Source: CAD feature listing. Evaluate the final solid. Frame: model axes, mm. A direction names the side the tool comes from. Coordinates: 2 decimals unless noted, no trailing zeros. Order: outer loops, then holes, each group sorted by start corner. A loop starts at its lowest first (then second) coordinate and runs counter-clockwise, first axis right, second up. Notation, with made-up numbers: (80.5, 41) - (102.5, 41) arc R12 ccw to (102.5, 45) - close; hole circle Ø4 at (-29.5, -17.75). An arc over 180 degrees is marked (long way). One line per question, with ' | ' between items. Start each with the question number.
(1) Access query for faces 4 (the flat face through (185, -10, -69.85)), 5 (the flat face through (-148, 44, -50.8)), 6 (the flat face through (185, -10, 120.65)), 7 (the flat face through (-4, 0, -2)). Directions: +Z, -Z, +X, -X, +Y, -Y. A direction counts if a zero-diameter tool reaches every point of the face in a straight line with its end or side. Return the directions, or none.
(2) Section D-D (z = -1). Return the cut outline in (x, y).
(3) Section A-A (x = -103). Return the cut outline in (y, z), then the cut area to 3 significant figures.
(4) Contact query for flat-ended pins moving along their axis: P1, Ø20.5, axis at x = -181.5, y = -13.5, coming from the -Z side; P2, Ø6.5, axis at y = 43.5, z = 3.5, coming from the -X side; P3, Ø2, axis at x = -176.5, z = 96.5, coming from the -Y side. Output: stop coordinate, or through.
(5) Section B-B (z = -88). Return the cut outline in (x, y), then the cut area to 3 significant figures.
(6) Draft query along Y for faces 1 (the cylindrical face through (-184.974, -25.395, -94.894)), 2 (the flat face through (-25.4, 45, -1)), 3 (the flat face through (-185, -10, 69.85)). Return one class per face: +Y half, -Y half, draft (parallel to the pull), parting line (faces both ways), or undercut.
(7) Line query: line 1 along Y through (x, z) = (-208, 36); line 2 along Y through (x, z) = (-63, -69.5); line 3 along Z through (x, y) = (-187.5, -12.5). Output: solid intervals per line, ascending.
(8) Section C-C (x = 210). Return the cut outline in (y, z).
from build123d import *

# Parameters (mm, degrees)
CHASIS_W                = 533.4
CHASIS_H                = 279.4
BOSS_EXTRUDE1_DEPTH     = 152.4
SKETCH3_W               = 63.5
SKETCH3_H               = 50.8
MIRROR2_COPY_1_SKETCH_W = 63.5
MIRROR2_COPY_1_SKETCH_H = 50.8
SKETCH4_W               = 101.6
SKETCH4_H               = 12.7
CUT_EXTRUDE1_DEPTH      = 241.3


with BuildPart() as part:
    # Chasis → Boss-Extrude1 (new body)
    with BuildSketch(Plane(origin=(0, 0, 0), x_dir=(1, 0, 0), z_dir=(0, 1, 0))):
        Rectangle(CHASIS_W, CHASIS_H)
    extrude(amount=BOSS_EXTRUDE1_DEPTH)

    # Sketch3 → Revolve2 (revolve)
    with BuildSketch(Plane(origin=(0, 38.1, 0), x_dir=(-1, 0, 0), z_dir=(0, -1, 0))):
        with Locations((215.9, -95.25)):
            Rectangle(SKETCH3_W, SKETCH3_H)
    revolve2 = revolve(axis=Axis((-184.15, 38.1, 69.85), (0, 0, 1)))

    # Mirror1: Revolve2 across plane
    add(revolve2.mirror(Plane.XY))

    # Mirror2: Revolve2 across plane
    add(revolve2.mirror(Plane(origin=(0, 0, 0), x_dir=(0, 0, 1), z_dir=(1, 0, 0))))

    # Mirror2 copy 1 sketch → Mirror2 copy 1 (revolve)
    with BuildSketch(Plane.XZ.offset(-38.1)):
        with Locations((215.9, -95.25)):
            Rectangle(MIRROR2_COPY_1_SKETCH_W, MIRROR2_COPY_1_SKETCH_H)
    revolve(axis=Axis((184.15, 38.1, -69.85), (0, 0, -1)))

    # Sketch4 → Cut-Extrude1 (cut)
    with BuildSketch(Plane.ZY.offset(266.7)):
        with Locations((0, 44.45)):
            Rectangle(SKETCH4_W, SKETCH4_H)
    extrude(amount=-CUT_EXTRUDE1_DEPTH, mode=Mode.SUBTRACT)


solid = part.part
Response values:
1) face 4: +X, -X, -Y | face 5: -X | face 6: +Z, +X, -X, -Y | face 7: -Y
2) outline: (-266.7, 0) - (266.7, 0) - (266.7, 152.4) - (-266.7, 152.4) - (-266.7, 50.8) - (-25.4, 50.8) - (-25.4, 38.1) - (-266.7, 38.1) - close
3) outline: (0, -139.7) - (152.4, -139.7) - (152.4, 139.7) - (0, 139.7) - close; hole (38.1, -50.8) - (50.8, -50.8) - (50.8, 50.8) - (38.1, 50.8) - close | area: 41,300 mm²
4) P1: stops at z = -120.65 | P2: stops at x = -25.4 | P3: stops at y = -25.05
5) outline: (-266.7, 0) - (-234.95, 0) arc R63.5 ccw to (-133.35, 0) - (133.35, 0) arc R63.5 ccw to (234.95, 0) - (266.7, 0) - (266.7, 152.4) - (-266.7, 152.4) - close | area: 84,900 mm²
6) face 1: -Y half | face 2: undercut | face 3: draft
7) line 1: y = 0 to 38.1, 50.8 to 152.4 | line 2: y = 0 to 152.4 | line 3: z = -120.65 to -69.85, 69.85 to 120.65
8) outline: (-19.9, -120.65) - (0, -120.65) - (0, -139.7) - (152.4, -139.7) - (152.4, 139.7) - (0, 139.7) - (0, 120.65) - (-19.9, 120.65) - (-19.9, 69.85) - (0, 69.85) - (0, -69.85) - (-19.9, -69.85) - close
